The listing builds one solid part. Answer for the finished solid, in the listing's coordinates (mm). Round coordinates to 2 decimals unless told otherwise and drop trailing zeros. Order: outer loops, then holes, each group sorted by start corner. A loop starts at its lowest first (then second) coordinate and runs counter-clockwise, first axis right, second up. Notation, with made-up numbers: (48.5, 84) - (82.5, 84) arc R23 cw to (82.5, 103) - close; hole circle Ø1 at (-7, 54.5). An arc over 180 degrees is marked (long way). One line per item, written item: value. Start each with the question number.
1. Section C-C, the plane x = 104.5 is taken. Give the vertices of the cut face in (y, z).
2. For a pull along X with two mould halves and no side action, classify faces 1 (the cylindrical face through (-132.922, -1.479, -101.921)), 2 (the cylindrical face through (138.304, -1.479, 43.554)), 3 (the flat face through (-50, 0, 137)) as released by +X, released by -X, zero draft, split by the parting line, or undercut.
3. Section B-B, the plane y = -2.2 is taken. Count the separate pieces of the cut face and the enclosed holes in it, then the cut area to 3 significant figures.
4. Section A-A, the plane z = 0 is taken. Give the vertices of the cut face in (x, y), then the cut area to 3 significant figures.
5. A flat-ended cylindrical pin translates along its axis: P1, Ø9.5, axis at x = -118.21, z = -102.43, coming from the +Y side. Find the tip coordinate at first contact, or state that the pin passes through.
6. Straight lines are drawn through the part: line 1 (Z direction, x = 0, y = -0.8); line 2 (X direction, y = -1.2, z = -148.5); line 3 (Z direction, x = -10.5, y = -1.2). For each, find the intervals that lie inside material, in ascending order.
from build123d import *

# Parameters (mm, degrees)
F0_R            = 167.5
F0_R_2          = 145
F1_DEPTH        = 3
F2_R            = 3
F3_DEPTH        = 25
F3_COPIES_COUNT = 11


# Not quite as in the source:
# - a pattern or mirror of a feature is missing from the dataset's text; its kind, count and spacing are read off the source's solid


with BuildPart() as f1:
    # F0 (on Front) → F1 (new body)
    with BuildSketch(Plane.XZ):
        Circle(F0_R)
        Circle(F0_R_2, mode=Mode.SUBTRACT)
    extrude(amount=F1_DEPTH)

    # F2 (on face) → F3 (cut)
    with BuildSketch(Plane.XZ.offset(3)):
        with Locations((0, 156.4114242792)):
            Circle(F2_R)
    f3 = extrude(amount=-F3_DEPTH, mode=Mode.SUBTRACT)

    # F3_copies: F3 ×11 about axis
    f3_copies_axis = Axis((0, 0, 0), (0, 1, 0))
    for i in range(1, F3_COPIES_COUNT):
        add(f3.rotate(f3_copies_axis, i * 360 / F3_COPIES_COUNT), mode=Mode.SUBTRACT)


solid = f1.part
Answer list:
1. outline: (-3, -130.9) - (0, -130.9) - (0, -100.52) - (-3, -100.52) - close; (-3, 100.52) - (0, 100.52) - (0, 130.9) - (-3, 130.9) - close
2. face 1: split by the parting line
2. face 2: undercut
2. face 3: zero draft
3. separate pieces: 1
3. enclosed holes: 12
3. area: 21,800 mm²
4. outline: (-167.5, -3) - (-145, -3) - (-145, 0) - (-167.5, 0) - close; (145, -3) - (167.5, -3) - (167.5, 0) - (145, 0) - close
4. area: 135 mm²
5. P1: stops at y = 0
6. line 1: z = -167.5 to -145, 145 to 153.41, 159.41 to 167.5
6. line 2: x = -77.49 to -46.62, -41.51 to 41.51, 46.62 to 77.49
6. line 3: z = -167.17 to -144.62, 144.62 to 167.17
